The model under review builds one solid part; all positions refer to its coordinate system, in mm. Face numbers are marked on the shaded views. A direction names the side the tool comes from. Coordinates: 2 decimals unless noted, no trailing zeros. Order: outer loops, then holes, each group sorted by start corner. A loop starts at its lowest first (then second) coordinate and runs counter-clockwise, first axis right, second up. Notation, with made-up numbers: M 7.25,76.25 L 47.25,76.25 A9 ccw 47.25,87.25 Z; hole C -9,87.25 d2. An arc over 180 degrees is marked long. Answer in a Markdown table with one row per item.
Solid Edge part; units mm, degrees
sketch "Sketch1" plane through (0, 0, 0) normal (0, 0, 1) x (1, 0, 0)
  line L0 (11.5, -10) -> (11.5, 10)
  line L1 (11.5, 10) -> (-11.5, 10)
  line L2 (-11.5, 10) -> (-11.5, -10)
  line L3 (-11.5, -10) -> (11.5, -10)
extrude "Protrusion1" add sketch "Sketch1" along normal mid plane 1.6
sketch "Sketch2" plane through (0, 0, 0.8) normal (0, 0, 1) x (1, 0, 0)
  line L0 (7.5, -7.5) -> (7.5, 7.5)
  line L1 (7.5, 7.5) -> (-7.5, 7.5)
  line L2 (-7.5, 7.5) -> (-7.5, -7.5)
  line L3 (-7.5, -7.5) -> (7.5, -7.5)
extrude "ExtrudedCutout_1" add sketch "Sketch2" along normal blind 5
sketch "Sketch3" plane through (0, 0, 5.8) normal (0, 0, 1) x (1, 0, 0)
  line L0 (1, -3.25) -> (-1, -3.25)
  line L1 (-1, -3.25) -> (-1, -2.25)
  line L2 (-1, -2.25) -> (1, -2.25)
  line L3 (1, -2.25) -> (1, -3.25)
  line L4 (-5.125, -2.25) -> (5.125, -2.25)
  line L5 (5.125, -2.25) -> (5.125, 2.25)
  line L6 (5.125, 2.25) -> (-5.125, 2.25)
  line L7 (-5.125, 2.25) -> (-5.125, -2.25)
extrude "ExtrudedProtrusion_3" add sketch "Sketch3" along normal blind 3
sketch "Sketch4" plane through (0, 0, 5.8) normal (0, 0, 1) x (1, 0, 0)
  line L0 (1, -2.25) -> (1, -3.25)
  line L1 (1, -3.25) -> (-1, -3.25)
  line L2 (-1, -3.25) -> (-1, -2.25)
  line L3 (-5.125, -2.25) -> (-1, -2.25)
  line L4 (-5.125, 2.25) -> (-5.125, -2.25)
  line L5 (5.125, 2.25) -> (-5.125, 2.25)
  line L6 (5.125, -2.25) -> (5.125, 2.25)
  line L7 (1, -2.25) -> (5.125, -2.25)
  line L8 (1.875, -4.125) -> (1.875, -3.125)
  line L9 (1.875, -3.125) -> (6, -3.125)
  line L10 (6, -3.125) -> (6, 3.125)
  line L11 (6, 3.125) -> (-6, 3.125)
  line L12 (-6, 3.125) -> (-6, -3.125)
  line L13 (-6, -3.125) -> (-1.875, -3.125)
  line L14 (-1.875, -3.125) -> (-1.875, -4.125)
  line L15 (-1.875, -4.125) -> (1.875, -4.125)
extrude "ExtrudedProtrusion_4" add sketch "Sketch4" along normal blind 0.5
sketch "Sketch5" plane through (0, 0, 0.8) normal (0, 0, 1) x (1, 0, 0)
  circle A0 centre (-10, 6.25) radius 0.75
  circle A1 centre (10, 6.25) radius 0.75
  circle A2 centre (10, -6.25) radius 0.75
  circle A3 centre (-10, -6.25) radius 0.75
extrude "Cutout1" cut sketch "Sketch5" against normal up to vertex (1.6 mm away)
sketch "Sketch6" plane through (0, -0.5, 8.8) normal (0, 0, 1) x (1, 0, 0)
  line L0 (-3.4, 1.9) -> (-3.4, -0.9)
  line L1 (-3.4, -0.9) -> (-2.4, -0.9)
  line L2 (-2.4, -0.9) -> (-2.4, 1.9)
  line L3 (-2.4, 1.9) -> (-3.4, 1.9)
  line L4 (3.4, -0.9) -> (3.4, 1.9)
  line L5 (3.4, 1.9) -> (2.4, 1.9)
  line L6 (2.4, 1.9) -> (2.4, -0.9)
  line L7 (2.4, -0.9) -> (3.4, -0.9)
extrude "Cutout2" cut sketch "Sketch6" against normal up to vertex (3 mm away)
properties material "Polycarbonate"
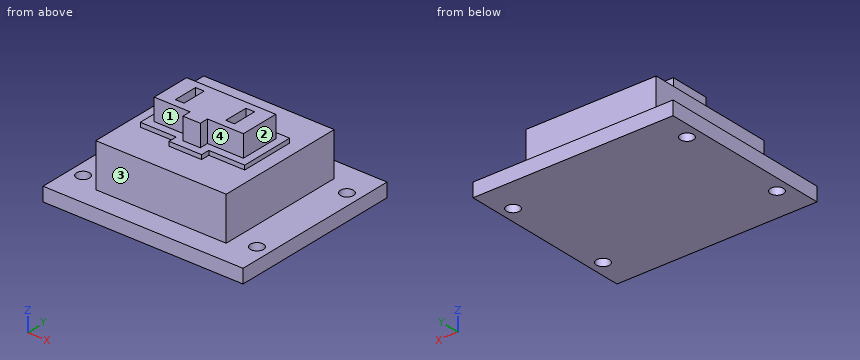
(1) Take a section at B-B (x = -10). Write out the cut boundary in (y, z).
Report:
| item | result |
|---|---|
| outline | M -10,-0.8 L -7,-0.8 L -7,0.8 L -10,0.8 Z; M -5.5,-0.8 L 5.5,-0.8 L 5.5,0.8 L -5.5,0.8 Z; M 7,-0.8 L 10,-0.8 L 10,0.8 L 7,0.8 Z |
(2) Take a section at A-A (y = -6.25). Write out the cut boundary in (x, z).
Report:
| item | result |
|---|---|
| outline | M -11.5,-0.8 L -10.75,-0.8 L -10.75,0.8 L -11.5,0.8 Z; M -9.25,-0.8 L 9.25,-0.8 L 9.25,0.8 L 7.5,0.8 L 7.5,5.8 L -7.5,5.8 L -7.5,0.8 L -9.25,0.8 Z; M 10.75,-0.8 L 11.5,-0.8 L 11.5,0.8 L 10.75,0.8 Z |
(3) Take a section at D-D (y = 3.5). Write out the cut boundary in (x, z), then the cut area to 3 significant figures.
Report:
| item | result |
|---|---|
| outline | M -11.5,-0.8 L 11.5,-0.8 L 11.5,0.8 L 7.5,0.8 L 7.5,5.8 L -7.5,5.8 L -7.5,0.8 L -11.5,0.8 Z |
| area | 112 mm^2 |
(4) Insertion check: P1, Ø2, axis at x = -3.5, z = 7.5, coming from the -Y side; P2, Ø1.1, axis at y = -2.5, z = 8, coming from the -X side (3 decimals); P3, Ø1.5, axis at x = 2, z = 2.5, coming from the -Y side. Each pin has a flat end and moves straight along its axis. Give the tip position at first contact, or say it passes through.
Report:
| item | result |
|---|---|
| P1 | y = -2.25 |
| P2 | x = -5.125 |
| P3 | y = -7.5 |
(5) Take a section at C-C (z = 0.5). Write out the cut boundary in (x, y).
Report:
| item | result |
|---|---|
| outline | M -11.5,-10 L 11.5,-10 L 11.5,10 L -11.5,10 Z; hole C -10,-6.25 d1.5; hole C -10,6.25 d1.5; hole C 10,-6.25 d1.5; hole C 10,6.25 d1.5 |
(6) Machinability: for the marked faces 1, 2, 3 and 4, which of the approach directions +Z, -Z, +X, -X, +Y, -Y give a long, thin tool a straight path to every point of the face, cutting with its end or side? Answer none if there is none.
Report:
| item | result |
|---|---|
| face 1 | +Z, -X, -Y |
| face 2 | +Z, +X, +Y, -Y |
| face 3 | +Z, +X, -X, -Y |
| face 4 | +Z, +X, -Y |
(7) To check wall thickness, follow line 1 (X direction, y = 1.25, z = 7.75) (3 decimals); line 2 (Y direction, x = -10, z = 0.15); line 3 (Z direction, x = 4.25, y = 4.25). State the ranges of each line that lie inside material, in increasing order. Write a range as [from, to].
Report:
| item | result |
|---|---|
| line 1 | [-5.125, -3.4], [-2.4, 2.4], [3.4, 5.125] |
| line 2 | [-10, -7], [-5.5, 5.5], [7, 10] |
| line 3 | [-0.8, 5.8] |
